Geometry: final body of the model. Coordinates: model frame, mm. Face numbers are marked on the shaded views. A direction names the side the tool comes from. Give positions to 0.01 mm unless a question says otherwise; leave off trailing zeros. Loops run counter-clockwise (first coordinate to the right, second up) from the corner with the lowest first, then second, coordinate; pieces in that order, holes last. Notation, with made-up numbers: (87.5, 88) -> (99.5, 88) arc R24 ccw to (99.5, 113) -> close; hole circle Ø6 at (40.25, 52). An arc over 180 degrees is marked (long way). Answer in a Markdown table with one row per item. Add a question column.
1) Line query: line 1 (X direction, y = -16, z = 4.75); line 2 (Y direction, x = -14, z = 3.75); line 3 (X direction, y = -14, z = 6). Output: solid intervals per line, ascending. Write a range as from..to.
2) Section query C-C (y = 29.5). Return the cut outline in (x, z), plus the area to 3 significant figures.
3) Draft query along X for the marked faces 6, 7, 8 and 9. Return one class per face: +X half, -X half, draft (parallel to the pull), parting line (faces both ways), or undercut.
4) First-contact query: P1, Ø9.5, axis at x = 18.5, y = 10.47, coming from the -Z side; P2, Ø2, axis at x = 2.5, z = 6, coming from the +Y side; P3, Ø4, axis at x = -29.5, z = 2, coming from the +Y side; P4, Ø1, axis at x = -27.5, y = 3.5, coming from the +Z side. Flat tips, straight axial feed; report the tip coordinate or a pass-through.
5) Access query for the marked faces 1, 2, 3, 4 and 5. Directions: +Z, -Z, +X, -X, +Y, -Y. A direction counts if a zero-diameter tool reaches every point of the face in a straight line with its end or side. Return the directions, or none.
6) Section query B-B (x = 0). Return the cut outline in (y, z), plus the area to 3 significant figures.
7) Section query D-D (x = -23.5). Return the cut outline in (y, z), plus the area to 3 significant figures.
8) Section query A-A (z = 1.75). Return the cut outline in (x, y).
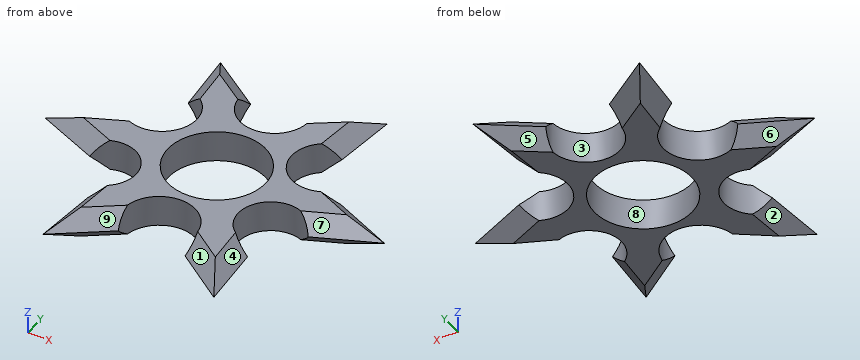
```python
from build123d import *

# Parameters (mm, degrees)
F0_R         = 11
F1_DEPTH     = 7
F2_SIZE      = 3.81
F3_T1_DEPTH  = 34.6394313852
F3_T3_DEPTH  = 34.3439110976
F4_SIZE      = 3.81
F5_T1_DEPTH  = 35.2279158768
F5_T3_DEPTH  = 35.1515641575
F5_T5_DEPTH  = 34.8076073963
F5_T7_DEPTH  = 34.8076073963
F5_T9_DEPTH  = 34.5979192148
F5_T11_DEPTH = 35.1515641575
F5_T13_DEPTH = 35.2279158768
F5_T15_DEPTH = 34.6394313852
F5_T17_DEPTH = 34.8076073963
F6_T1_DEPTH  = 29.7856896268


# Not quite as in the source:
# - a fillet or chamfer that OpenCascade refuses, or shapes differently, is made with other operations: its cross-section is extruded or revolved along the edge and cut away or added


with BuildPart() as f1:
    # F0 (on Top) → F1 (new body)
    with BuildSketch(Plane.XY):
        with BuildLine():
            Line((-19.3098304855, 33.4750442975), (-17.9191186068, 18.4962593726))
            ThreePointArc((-17.9191186068, 18.4962593726), (-12.1734101316, 6.7065768921), (-25.2838117957, 6.35))
            Line((-25.2838117957, 6.35), (-39.5676235915, 0))
            Line((-39.5676235915, 0), (-25.3535799067, -6.3189839441))
            ThreePointArc((-25.3535799067, -6.3189839441), (-12.9763127609, -6.8724869317), (-18.8926645602, -17.7582523592))
            Line((-18.8926645602, -17.7582523592), (-20.2989239466, -32.9044930863))
            Line((-20.2989239466, -32.9044930863), (-7.891724267, -24.1040629982))
            ThreePointArc((-7.891724267, -24.1040629982), (-0.2207247048, -12.9944902326), (7.1436805269, -24.3096295115))
            Line((7.1436805269, -24.3096295115), (19.2464965418, -33.1737534264))
            Line((19.2464965418, -33.1737534264), (19.2872961226, -33.1740312262))
            Line((19.2872961226, -33.1740312262), (18.113880894, -18.0395493303))
            ThreePointArc((18.113880894, -18.0395493303), (12.3636945983, -7.0651033251), (24.7479456966, -6.6998194754))
            Line((24.7479456966, -6.6998194754), (39.056406052, -0.5976429607))
            Line((39.056406052, -0.5976429607), (24.8707754105, 5.9687611329))
            ThreePointArc((24.8707754105, 5.9687611329), (11.7673092468, 6.524596873), (17.6915767021, 18.225572644))
            Line((17.6915767021, 18.225572644), (19.3098304855, 33.1814855899))
            Line((19.3098304855, 33.1814855899), (7.1525325905, 24.8331700857))
            ThreePointArc((7.1525325905, 24.8331700857), (0.2505296838, 13.6219778067), (-6.9026308059, 24.6746142094))
            Line((-6.9026308059, 24.6746142094), (-19.3098304855, 33.4750442975))
        make_face()
        Circle(F0_R, mode=Mode.SUBTRACT)
    extrude(amount=F1_DEPTH)

    # F2
    f2_edges = [f1.edges().sort_by_distance(p)[0] for p in [
        (18.500704, 25.703529, 7),
        (13.231182, 29.007328, 7),
    ]]
    chamfer(f2_edges, length=F2_SIZE)

    # F3: chamfer of 3.81 on 2 edges, made by hand

    # F3_s2 → F3_t1 (cut)
    with BuildSketch(Plane(origin=(1.0999249917, 10.1655145758, 0), x_dir=(0, 0, 1), z_dir=(0.1075737229, 0.9941971103, 0))):
        Polygon((3.81, 15.6283217323), (0, 11.8183217323), (0, 15.6283217323), align=None)
    extrude(amount=F3_T1_DEPTH, mode=Mode.SUBTRACT)

    # F3_s4 → F3_t3 (cut)
    with BuildSketch(Plane(origin=(36.6832724438, 25.190098551, 0), x_dir=(0, 0, 1), z_dir=(-0.8243528709, -0.5660762706, 0))):
        Polygon((0, 12.6124160802), (3.81, 16.4224160802), (0, 16.4224160802), align=None)
    extrude(amount=F3_T3_DEPTH, mode=Mode.SUBTRACT)

    # F4 (call 1 of 6: OpenCascade refuses the feature's edges together)
    f4_edges = [f1.edges().sort_by_distance(p)[0] for p in [
        (31.902176, -3.648731, 7),
        (31.963591, 2.685559, 7),
    ]]
    chamfer(f4_edges, length=F4_SIZE)

    # F4#2 (call 2 of 6)
    f4_2_edges = [f1.edges().sort_by_distance(p)[0] for p in [
        (18.700589, -25.60679, 7),
    ]]
    chamfer(f4_2_edges, length=F4_SIZE)

    # F4#3 (call 3 of 6)
    f4_3_edges = [f1.edges().sort_by_distance(p)[0] for p in [
        (13.195089, -28.741691, 7),
    ]]
    chamfer(f4_3_edges, length=F4_SIZE)

    # F4#4 (call 4 of 6)
    f4_4_edges = [f1.edges().sort_by_distance(p)[0] for p in [
        (-14.095324, -28.504278, 7),
        (-19.595794, -25.331373, 7),
    ]]
    chamfer(f4_4_edges, length=F4_SIZE)

    # F4#5 (call 5 of 6)
    f4_5_edges = [f1.edges().sort_by_distance(p)[0] for p in [
        (-32.460602, -3.159492, 7),
        (-32.425718, 3.175, 7),
    ]]
    chamfer(f4_5_edges, length=F4_SIZE)

    # F4#6 (call 6 of 6)
    f4_6_edges = [f1.edges().sort_by_distance(p)[0] for p in [
        (-18.614475, 25.985652, 7),
        (-13.106231, 29.074829, 7),
    ]]
    chamfer(f4_6_edges, length=F4_SIZE)

    # F5: chamfer of 3.81 on 9 edges, made by hand

    # F5_s2 → F5_t1 (cut)
    with BuildSketch(Plane(origin=(41.2840936669, -19.1100451228, 0), x_dir=(0, 0, 1), z_dir=(-0.9074917218, 0.4200699643, 0))):
        Polygon((0, 12.0540670557), (3.81, 15.8640670557), (0, 15.8640670557), align=None)
    extrude(amount=F5_T1_DEPTH, mode=Mode.SUBTRACT)

    # F5_s4 → F5_t3 (cut)
    with BuildSketch(Plane(origin=(9.5091795604, 4.0554113263, 0), x_dir=(0, 0, 1), z_dir=(0.9198423531, 0.3922882173, 0))):
        Polygon((0, 12.0611052097), (3.81, 15.8711052097), (0, 15.8711052097), align=None)
    extrude(amount=F5_T3_DEPTH, mode=Mode.SUBTRACT)

    # F5_s6 → F5_t5 (cut)
    with BuildSketch(Plane(origin=(-37.0237803275, -26.260977399, 0), x_dir=(0, 0, 1), z_dir=(0.8156523083, 0.5785424029, 0))):
        Polygon((0, 11.2848375041), (3.81, 15.0948375041), (0, 15.0948375041), align=None)
    extrude(amount=F5_T5_DEPTH, mode=Mode.SUBTRACT)

    # F5_s8 → F5_t7 (cut)
    with BuildSketch(Plane(origin=(-0.8903351992, -9.5894337742, 0), x_dir=(0, 0, 1), z_dir=(-0.0924478322, -0.9957175294, 0))):
        Polygon((0, 13.3600453443), (3.81, 17.1700453443), (0, 17.1700453443), align=None)
    extrude(amount=F5_T7_DEPTH, mode=Mode.SUBTRACT)

    # F5_s10 → F5_t9 (cut)
    with BuildSketch(Plane(origin=(8.3331341524, -6.1032022329, 0), x_dir=(0, 0, 1), z_dir=(0.806763245, -0.5908748315, 0))):
        Polygon((0, 11.5810945617), (3.81, 15.3910945617), (0, 15.3910945617), align=None)
    extrude(amount=F5_T9_DEPTH, mode=Mode.SUBTRACT)

    # F5_s12 → F5_t11 (cut)
    with BuildSketch(Plane(origin=(-41.9914373351, 18.6676799506, 0), x_dir=(0, 0, 1), z_dir=(0.9137726258, -0.406226031, 0))):
        Polygon((0, 12.2633986894), (3.81, 16.0733986894), (0, 16.0733986894), align=None)
    extrude(amount=F5_T11_DEPTH, mode=Mode.SUBTRACT)

    # F5_s14 → F5_t13 (cut)
    with BuildSketch(Plane(origin=(-9.8011321421, -4.357183502, 0), x_dir=(0, 0, 1), z_dir=(-0.9137726258, -0.406226031, 0))):
        Polygon((3.81, 16.0733986894), (0, 12.2633986894), (0, 16.0733986894), align=None)
    extrude(amount=F5_T13_DEPTH, mode=Mode.SUBTRACT)

    # F5_s16 → F5_t15 (cut)
    with BuildSketch(Plane(origin=(-4.1522899993, 44.7226055925, 0), x_dir=(0, 0, 1), z_dir=(0.0924478322, -0.9957175294, 0))):
        Polygon((3.81, 16.1324414242), (0, 12.3224414242), (0, 16.1324414242), align=None)
    extrude(amount=F5_T15_DEPTH, mode=Mode.SUBTRACT)

    # F5_s18 → F5_t17 (cut)
    with BuildSketch(Plane(origin=(-8.2440794116, 5.8475277562, 0), x_dir=(0, 0, 1), z_dir=(-0.8156523083, 0.5785424029, 0))):
        Polygon((0, 12.3224414242), (3.81, 16.1324414242), (0, 16.1324414242), align=None)
    extrude(amount=F5_T17_DEPTH, mode=Mode.SUBTRACT)

    # F6: chamfer of 3.81 on 1 edges, made by hand

    # F6_s2 → F6_t1 (cut)
    with BuildSketch(Plane(origin=(3.0435836487, -39.2555512393, 0), x_dir=(0, 0, 1), z_dir=(-0.0773005765, 0.9970078339, 0))):
        Polygon((0, 12.8552135911), (3.81, 16.6652135911), (0, 16.6652135911), align=None)
    extrude(amount=F6_T1_DEPTH, mode=Mode.SUBTRACT)


solid = f1.part
```
Evaluation:
| question | item | result |
|---|---|---|
| 1 | line 1 | -14.57..-6.64, 5.98..13.58 |
| 1 | line 2 | -27.75..-15.45, -5.48..4.64, 16.87..29.02 |
| 1 | line 3 | -12.94..-4.25, 3.59..12.12 |
| 2 | outline | (-18.63, 3.5) -> (-17.02, 1.89) -> (-14.24, 3.5) -> (-17.02, 5.11) -> close; (14.5, 3.5) -> (17.11, 2.02) -> (18.6, 3.5) -> (17.11, 4.98) -> close |
| 2 | area | 13.1 mm² |
| 3 | face 6 | -X half |
| 3 | face 7 | +X half |
| 3 | face 8 | undercut |
| 3 | face 9 | undercut |
| 4 | P1 | through |
| 4 | P2 | y = 14.37 |
| 4 | P3 | y = 4.72 |
| 4 | P4 | z = 5.39 |
| 5 | face 1 | +Z, -Y |
| 5 | face 2 | -Z, -X |
| 5 | face 3 | +Z, -Z |
| 5 | face 4 | +Z, +X |
| 5 | face 5 | -Z, +Y |
| 6 | outline | (-13, 0) -> (-11, 0) -> (-11, 7) -> (-13, 7) -> close; (11, 0) -> (13.62, 0) -> (13.62, 7) -> (11, 7) -> close |
| 6 | area | 32.4 mm² |
| 7 | outline | (-4.46, 1.36) -> (-2.97, 0) -> (2.97, 0) -> (4.49, 1.39) -> (4.49, 5.61) -> (2.97, 7) -> (-2.97, 7) -> (-4.46, 5.64) -> close |
| 7 | area | 58.5 mm² |
| 8 | outline | (-34.5, 0) -> (-23.86, -4.73) arc R7.31 cw (long way) to (-16.78, -17.31) -> (-17.83, -28.63) -> (-8.42, -21.95) arc R8.13 cw (long way) to (7.73, -22.18) -> (16.89, -28.89) -> (16.01, -17.56) arc R7.31 cw (long way) to (23.28, -5.09) -> (33.99, -0.52) -> (23.38, 4.39) arc R7.8 cw (long way) to (15.56, 17.69) -> (16.78, 28.94) -> (7.82, 22.79) arc R7.78 cw (long way) to (-7.53, 22.59) -> (-16.84, 29.2) -> (-15.8, 17.93) arc R7.8 cw (long way) to (-23.82, 4.75) -> close; hole circle Ø22 at (0, 0) |
